Check sheet for the drawn part. Datum: minimum x, y, z corner. Units: mm. A direction names the side the tool comes from. Give positions to 0.01 mm unless a question says otherwise; leave off trailing zeros. Loops run counter-clockwise (first coordinate to the right, second up) from the corner with the lowest first, then second, coordinate; pieces in that order, holes last. Notation, with made-up numbers: (64, 7) - (92, 7) arc R33 cw to (92, 46) - close; hole circle Ø7 at (-2.5, 54). An arc over 180 degrees is marked (long way). Use one line per item in the form item = value.
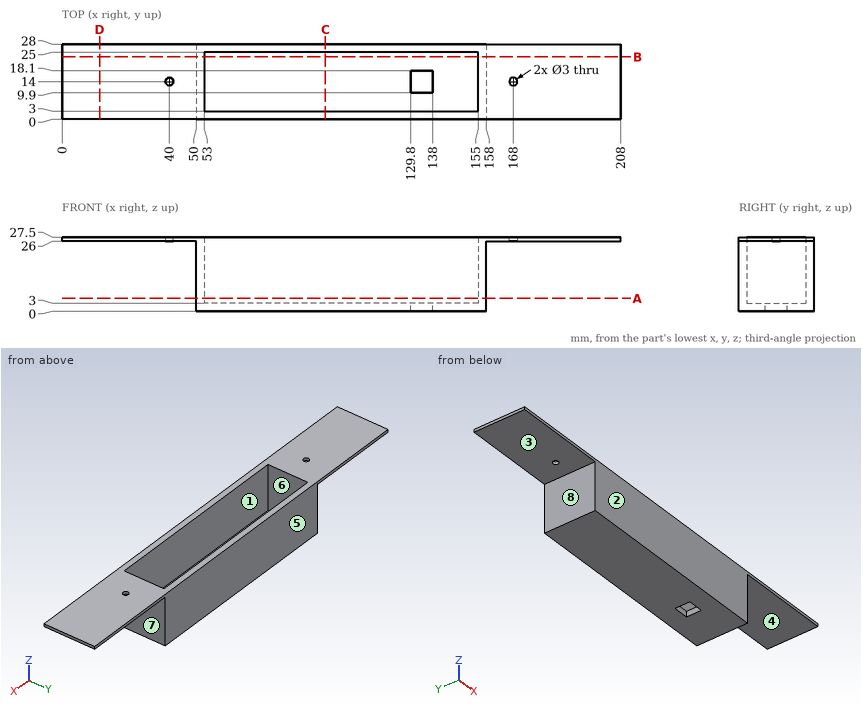
Item 1: Section check D-D on x = 14. Record the boundary of the cut face in (y, z).
Answer block:
outline = (0, 26) - (28, 26) - (28, 27.5) - (0, 27.5) - close
Item 2: Thickness scan on L1, parallel to Y at x = 40, z = 26.8; L2, parallel to Y at x = 87, z = 5.5; L3, parallel to X at y = 6, z = 21. Record the ranges inside material, lowest first.
Answer block:
L1 = 0 to 12.5, 15.5 to 28
L2 = 0 to 3, 25 to 28
L3 = 50 to 53, 155 to 158
Item 3: Mould release check, pull along X, two halves, no side actions. Record for the marked faces 5, 6, 7 and 8: released by +X, released by -X, zero draft, split by the parting line, or undercut.
Answer block:
face_5 = zero draft
face_6 = undercut
face_7 = released by +X
face_8 = released by -X
Item 4: Access from +Z, -Z, +X, -X, +Y, -Y to the whole of each face (thin tool, end or side, straight path). Record for the marked faces 1, 2, 3 and 4.
Answer block:
face_1 = +Z
face_2 = +Z, -Z, +X, -X, -Y
face_3 = -Z, -X, +Y, -Y
face_4 = -Z, +X, +Y, -Y
Item 5: Section check A-A on z = 4.75. Record the boundary of the cut face in (x, y), then the cut area to 3 significant figures.
Answer block:
outline = (50, 0) - (158, 0) - (158, 28) - (50, 28) - close; hole (53, 3) - (155, 3) - (155, 25) - (53, 25) - close
area = 780 mm2
Item 6: Gauge pin test, flat ends, axial feed: P1, Ø2.5, axis at y = 15.5, z = 2, coming from the -X side; P2, Ø12, axis at x = 21.5, y = 11, coming from the -Z side; P3, Ø3, axis at y = 19, z = 6.5, coming from the +X side. Record the tip position at first contact, or that the pin passes through.
Answer block:
P1 = 50
P2 = 26
P3 = 158
Item 7: Section check B-B on y = 23.25. Record the boundary of the cut face in (x, z).
Answer block:
outline = (0, 26) - (50, 26) - (50, 0) - (158, 0) - (158, 26) - (208, 26) - (208, 27.5) - (155, 27.5) - (155, 3) - (53, 3) - (53, 27.5) - (0, 27.5) - close
Item 8: Section check C-C on x = 98. Record the boundary of the cut face in (y, z).
Answer block:
outline = (0, 0) - (28, 0) - (28, 27.5) - (25, 27.5) - (25, 3) - (3, 3) - (3, 27.5) - (0, 27.5) - close
